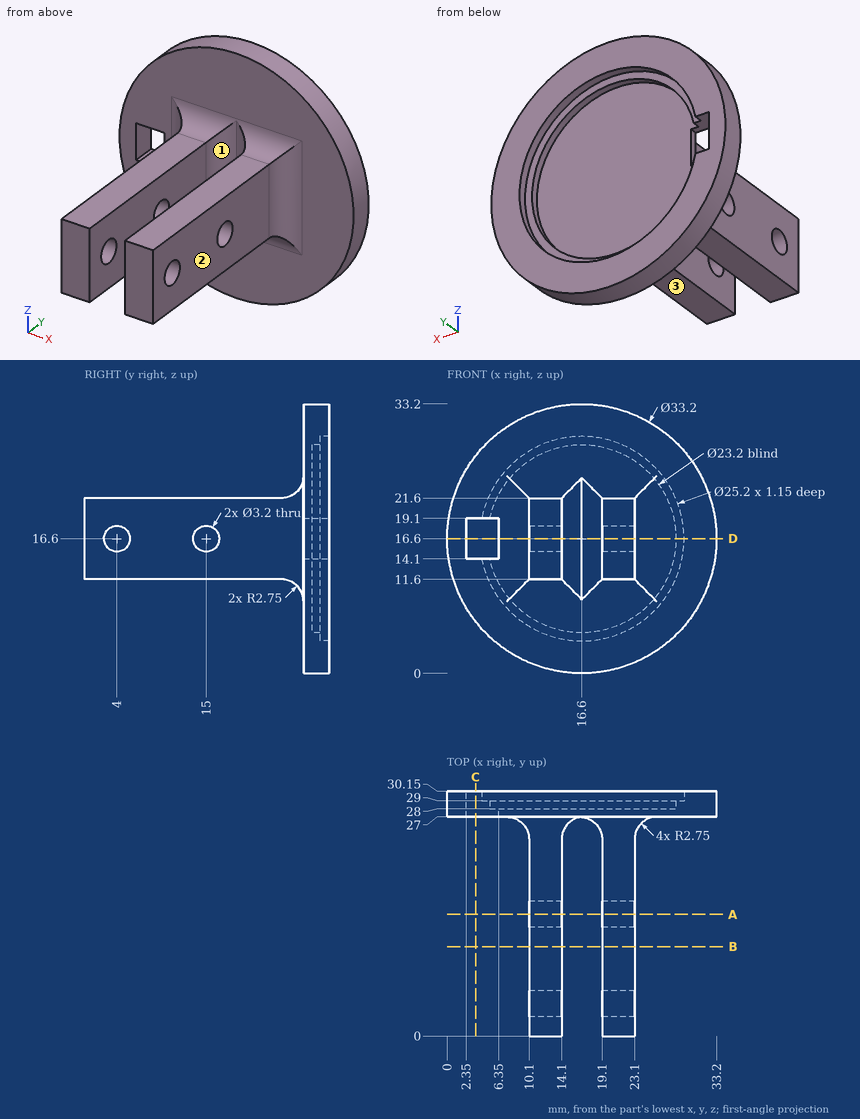
Check sheet for the drawn part. Datum: minimum x, y, z corner. Units: mm. A direction names the side the tool comes from. Round coordinates to 2 decimals unless told otherwise and drop trailing zeros. Loops run counter-clockwise (first coordinate to the right, second up) from the corner with the lowest first, then second, coordinate; pieces in that order, holes last.
Item 1: Cross-section at C-C on x = 3.5. Record the boundary of the cut face in (y, z), then the cut area to 3 significant figures.
Item 2: Gauge pin test, flat ends, axial feed: pin 1 (11 mm diameter, centred on y = 11.5, z = 18, fed in from +X); pin 2 (1.2 mm diameter, centred on x = 20.5, y = 9.5, fed in from -Z); pin 3 (5 mm diameter, centred on y = 9, z = 15.5, fed in from -X). Record the tip position at first contact, or that the pin passes through.
Item 3: Access from +Z, -Z, +X, -X, +Y, -Y to the whole of each face (thin tool, end or side, straight path). Record for the marked faces 1, 2 and 3.
Item 4: Cross-section at B-B on y = 11. Record the boundary of the cut face in (x, z), then the cut area to 3 significant figures.
Item 5: Thickness scan on line 1 (Z direction, x = 16.6, y = 29.75); line 2 (X direction, y = 5.5, z = 21); line 3 (X direction, y = 29.5, z = 16.6). Record the ranges inside material, lowest first.
Item 6: Cross-section at A-A on y = 15. Record the boundary of the cut face in (x, z).
Item 7: Cross-section at D-D on z = 16.6. Count the separate pieces of the cut face and the enclosed holes in it, then the cut area to 3 significant figures.
Answer sheet:
1. outline: (27, 6.4) - (30.15, 6.4) - (30.15, 14.1) - (27, 14.1) - close; (27, 19.1) - (30.15, 19.1) - (30.15, 26.8) - (27, 26.8) - close
1. area: 48.5 mm2
2. pin 1: stops at x = 23.1
2. pin 2: stops at z = 11.6
2. pin 3: stops at x = 10.1
3. face 1: +Z, -Z, -Y
3. face 2: +Z, -Z, +X, -Y
3. face 3: -Z, +X, -X, -Y
4. outline: (10.1, 11.6) - (14.1, 11.6) - (14.1, 21.6) - (10.1, 21.6) - close; (19.1, 11.6) - (23.1, 11.6) - (23.1, 21.6) - (19.1, 21.6) - close
4. area: 80.0 mm2
5. line 1: z = 0 to 4, 29.2 to 33.2
5. line 2: x = 10.1 to 14.1, 19.1 to 23.1
5. line 3: x = 0 to 2.35, 29.2 to 33.2
6. outline: (10.1, 11.6) - (14.1, 11.6) - (14.1, 15) - (10.1, 15) - close; (10.1, 18.2) - (14.1, 18.2) - (14.1, 21.6) - (10.1, 21.6) - close; (19.1, 11.6) - (23.1, 11.6) - (23.1, 15) - (19.1, 15) - close; (19.1, 18.2) - (23.1, 18.2) - (23.1, 21.6) - (19.1, 21.6) - close
7. separate pieces: 6
7. enclosed holes: 0
7. area: 215 mm2
